Read the model definition and answer for the solid it produces. Units are mm, in the model's axes. Coordinates: 2 decimals unless noted, no trailing zeros. Loops run counter-clockwise (first coordinate to the right, second up) from the corner with the lowest first, then second, coordinate; pieces in that order, holes last. Notation, with made-up numbers: (23.5, 80.25) - (72.5, 80.25) arc R17 ccw to (72.5, 91.25) - close; hole circle Ø7 at (88.25, 87). An arc over 180 degrees is marked (long way). Use one line per item in the form item = value.
from build123d import *

# Parameters (mm, degrees)
BASPROSKE_W        = 12
BASPROSKE_H        = 9
TOOTHCUT_DEPTH     = 18.492855685
TEETHCUTS_COUNT    = 10
TEETHCUTS_ANGLE    = 324
BORSKE_R           = 2
BORE_DEPTH         = 50.0000508
CUT_EXTRUDE1_DEPTH = 18


with BuildPart() as part:
    # BasProSke → Base-Revolve (revolve)
    with BuildSketch(Plane(origin=(0, 0, 0), x_dir=(1, 0, 0), z_dir=(0, 1, 0)), mode=Mode.PRIVATE) as base_revolve_sk:
        with Locations((6, 4.5)):
            Rectangle(BASPROSKE_W, BASPROSKE_H)
    revolve(base_revolve_sk.sketch.rotate(Axis((-10, 0, 0), (1, 0, 0)), 180), axis=Axis((-10, 0, 0), (1, 0, 0)))

    # TooCutSke → ToothCut (cut, through all)
    with BuildSketch(Plane(origin=(0, 0, 0), x_dir=(0, 0, -1), z_dir=(1, 0, 0))):
        with BuildLine():
            ThreePointArc((0.883878355, 5.554109745), (0, 5.624), (-0.883878355, 5.554109745))
            ThreePointArc((-0.883878355, 5.554109745), (-1.258245767, 7.379188248), (-2.637816971, 8.631324741))
            ThreePointArc((-2.637816971, 8.631324741), (0, 9.0254), (2.637816971, 8.631324741))
            ThreePointArc((2.637816971, 8.631324741), (1.258245767, 7.379188248), (0.883878355, 5.554109745))
        make_face()
    toothcut = extrude(amount=TOOTHCUT_DEPTH, mode=Mode.SUBTRACT)

    # TeethCuts: ToothCut ×10 about axis
    teethcuts_axis = Axis((-10, 0, 0), (1, 0, 0))
    for i in range(1, TEETHCUTS_COUNT):
        add(toothcut.rotate(teethcuts_axis, i * TEETHCUTS_ANGLE / (TEETHCUTS_COUNT - 1)), mode=Mode.SUBTRACT)

    # BorSke → Bore (cut, symmetric)
    with BuildSketch(Plane(origin=(0, 0, 0), x_dir=(0, 0, -1), z_dir=(1, 0, 0))):
        with Locations(Location((0, 0, 0), (0, 0, 180))):
            Circle(BORSKE_R)
    extrude(amount=BORE_DEPTH, both=True, mode=Mode.SUBTRACT)

    # Sketch1 → Cut-Extrude1 (cut)
    with BuildSketch(Plane(origin=(12, 0, 0), x_dir=(0, 0, -1), z_dir=(1, 0, 0))):
        with BuildLine():
            Line((2, 1.5), (2, -1.5))
            ThreePointArc((2, -1.5), (-2.5, 0), (2, 1.5))
        make_face()
    extrude(amount=-CUT_EXTRUDE1_DEPTH, mode=Mode.SUBTRACT)


solid = part.part
Item 1: The part is cut by section A-A on z = 0. Give the vertices of the cut face in (x, y).
Results below:
outline = (0, -5.62) - (12, -5.62) - (12, -2.5) - (0, -2.5) - close; (0, 2.5) - (12, 2.5) - (12, 5.62) - (0, 5.62) - close
Item 2: The part is cut by section C-C on z = 4.5. Give the vertices of the cut face in (x, y), plus the area to 3 significant figures.
Results below:
outline = (0, -4.65) - (12, -4.65) - (12, 4.65) - (0, 4.65) - close
area = 112 mm²
Item 3: The part is cut by section D-D on y = 3.5. Give the vertices of the cut face in (x, z), plus the area to 3 significant figures.
Results below:
outline = (0, -6.65) - (12, -6.65) - (12, 6.65) - (0, 6.65) - close
area = 160 mm²
Item 4: For a pull along Y with two mould halves and no side action, classify faces 1 (the cylindrical face through (5.916, -3.444, 6.598)), 2 (the cylindrical face through (5.916, -1.082, 7.414)) as +Y half, -Y half, draft (parallel to the pull), parting line (faces both ways), or undercut.
Results below:
face_1 = undercut
face_2 = undercut
Item 5: The part is cut by section B-B on y = -0.5. Give the vertices of the cut face in (x, z), plus the area to 3 significant figures.
Results below:
outline = (0, -8.66) - (12, -8.66) - (12, -2) - (0, -2) - close; (0, 2.45) - (12, 2.45) - (12, 8.66) - (0, 8.66) - close
area = 154 mm²
Item 6: Each of these flat-tipped pins is pushed along its axis until it touches: P1, Ø3, axis at y = 0, z = 0, coming from the -X side; P2, Ø4, axis at x = 10.5, z = 0.5, coming from the -Y side; P3, Ø1, axis at x = 10.5, z = -3.5, coming from the -Y side; P4, Ø2, axis at x = 8, z = -6, coming from the -Y side. Where does it stop, or does it pass through?
Results below:
P1 = through
P2 = -8.57
P3 = -8.42
P4 = -5.5
Item 7: Find the intervals of material crossed by L1, parallel to Z at x = 8, y = 0; L2, parallel to Y at x = 3.25, z = 0; L3, parallel to Y at x = 3.75, z = 3, in increasing order.
Results below:
L1 = -9 to -2, 2.5 to 9
L2 = -5.62 to -2.5, 2.5 to 5.62
L3 = -8.42 to -5.66, -4.76 to 4.76, 5.66 to 8.42
